from build123d import *

# Parameters (mm, degrees)
SKETCH2_R           = 30
CUT_EXTRUDE1_DEPTH  = 1031.526551259
SKETCH3_R           = 25
BOSS_EXTRUDE1_DEPTH = 1270
SKETCH4_R           = 12
CUT_EXTRUDE2_DEPTH  = 1103.63
CUT_EXTRUDE3_START  = -1016
SKETCH5_R           = 25
SKETCH5_R_2         = 20
CUT_EXTRUDE3_DEPTH  = 1016
BOSS_EXTRUDE2_DEPTH = 304.8
FILLET1_R           = 19.05


with BuildPart() as part:
    # Sketch1 → Revolve1 (revolve)
    with BuildSketch(Plane(origin=(0, 0, 0), x_dir=(0, 0, -1), z_dir=(1, 0, 0)), mode=Mode.PRIVATE) as revolve1_sk:
        with BuildLine():
            Line((-966.206657789, 37.7), (-966.206657789, 25))
            Line((-966.206657789, 25), (0, 25))
            Line((0, 25), (0, 0))
            Line((0, 0), (1016, 0))
            ThreePointArc((1016, 0), (980.290458762, 86.210458762), (894.08, 121.92))
            Line((894.08, 121.92), (0, 121.92))
            add(Edge.make_bspline(
                [(0, 121.92), (-738.002228528, 121.92), (-966.206657789, 37.7)],
                knots=[1.570796327, 1.570796327, 1.570796327, 2.827220811, 2.827220811, 2.827220811], degree=2, weights=[1, 0.809079465, 1]))
        make_face()
    revolve(revolve1_sk.sketch.rotate(Axis((0, 0, 0), (0, 0, -1)), 90), axis=Axis((0, 0, 0), (0, 0, -1)))

    # Sketch2 → Cut-Extrude1 (cut, through all)
    with BuildSketch(Plane.XY):
        with Locations(Location((0, 0, 0), (0, 0, 180))):
            Circle(SKETCH2_R)
    extrude(amount=CUT_EXTRUDE1_DEPTH, mode=Mode.SUBTRACT)

    # Sketch3 → Boss-Extrude1 (add)
    with BuildSketch(Plane.XY):
        with Locations(Location((0, 0, 0), (0, 0, 180))):
            Circle(SKETCH3_R)
    extrude(amount=BOSS_EXTRUDE1_DEPTH)

    # Sketch4 → Cut-Extrude2 (cut)
    with BuildSketch(Plane.XY.offset(1270)):
        Circle(SKETCH4_R)
    extrude(amount=-CUT_EXTRUDE2_DEPTH, mode=Mode.SUBTRACT)

    # Sketch5 → Cut-Extrude3 (cut)
    with BuildSketch(Plane.XY.offset(1079.5).offset(CUT_EXTRUDE3_START)):
        with Locations(Location((0, 0, 0), (0, 0, 180))):
            Circle(SKETCH5_R)
        Circle(SKETCH5_R_2, mode=Mode.SUBTRACT)
    extrude(amount=CUT_EXTRUDE3_DEPTH, mode=Mode.SUBTRACT)

    # Sketch6 → Boss-Extrude2 (add)
    with BuildSketch(Plane.XY):
        with BuildLine():
            Line((-25.4, 170.044817078), (25.4, 170.044817078))
            Line((25.4, 170.044817078), (25.4, 119.244817078))
            ThreePointArc((25.4, 119.244817078), (0, 121.92), (-25.4, 119.244817078))
            Line((-25.4, 119.244817078), (-25.4, 170.044817078))
        make_face()
    extrude(amount=-BOSS_EXTRUDE2_DEPTH)

    # Fillet1
    fillet1_edges = [part.edges().sort_by_distance(p)[0] for p in [
        (-25.4, 144.644817078, -304.8),
        (25.4, 144.644817078, -304.8),
        (-25.4, 144.644817078, 0),
        (25.4, 144.644817078, 0),
    ]]
    fillet(fillet1_edges, radius=FILLET1_R)


solid = part.part
Source: CAD feature listing. Evaluate the final solid. Frame: model axes, mm. A direction names the side the tool comes from. Round coordinates to 2 decimals unless told otherwise and drop trailing zeros. Loops run counter-clockwise (first coordinate to the right, second up) from the corner with the lowest first, then second, coordinate; pieces in that order, holes last.
Q1. Section B-B, the plane z = -796. Return loops of the section in (x, y).
Q2. Section A-A, the plane z = 605.5. State how many separate pieces and enclosed holes the cut face has, plus the area to 3 significant figures.
Q3. Access query for faces 1 (the face through (-4.336, -19.524, 564.388)), 2 (the face through (6, 11, 1270)), 3 (the face through (-23.846, -7.509, 31.306)), 4 (the face through (-25.4, 144, -151)). Directions: +Z, -Z, +X, -X, +Y, -Y. A direction counts if a zero-diameter tool reaches every point of the face in a straight line with its end or side. Return the directions, or none.
Q4. Mould query, pull axis Y, two halves, no side actions, for faces 5 (the face through (7, -25, 0)), 6 (the face through (25.4, 145, -151)), 7 (the face through (0, 170.045, -150)). Classes: pulls with the +Y half, pulls with the -Y half, needs draft (parallel to the pull), parting line crosses it, or undercut.
Q5. Ray query, line 1 (Y direction, x = 0, z = 962.5); line 2 (Y direction, x = 0, z = 354); line 3 (Y direction, x = -13.5, z = 921). Return the intervals inside material, ascending.
Q6. First-contact query: P1, Ø1.5, axis at x = 23, y = -19, coming from the -Z side; P2, Ø10, axis at y = -74.5, z = -170, coming from the -X side; P3, Ø4, axis at y = 23.5, z = -619, coming from the -X side. Flat tips, straight axial feed; report the tip coordinate or a pass-through.
Solutions:
1. outline: circle Ø243.84 at (0, 0)
2. separate pieces: 2
2. enclosed holes: 2
2. area: 28,100 mm2
3. face 1: none
3. face 2: +Z, +X, -X, +Y, -Y
3. face 3: +Z
3. face 4: +Z, -Z, -X, +Y
4. face 5: undercut
4. face 6: needs draft
4. face 7: pulls with the +Y half
5. line 1: y = -39.04 to -30, -20 to -12, 12 to 20, 30 to 39.04
5. line 2: y = -114.28 to -30, -20 to -12, 12 to 20, 30 to 114.28
5. line 3: y = -49.67 to -26.79, -14.76 to 14.76, 26.79 to 49.67
6. P1: stops at z = -1012.48
6. P2: stops at x = -100.17
6. P3: stops at x = -120.01
